from build123d import *

# Parameters (mm, degrees)
F0_R     = 38.1
F1_DEPTH = 2235.2
F2_R     = 38.1
F2_R_2   = 12.7
F3_DEPTH = 101.6
F4_R     = 38.1
F4_R_2   = 12.7
F5_DEPTH = 101.6


with BuildPart() as f1:
    # F0 (on Front) → F1 (new body)
    with BuildSketch(Plane.XZ):
        Circle(F0_R)
    extrude(amount=F1_DEPTH)

    # F2 (on face) → F3 (cut)
    with BuildSketch(Plane.XZ.offset(2235.2)):
        Circle(F2_R)
        Circle(F2_R_2, mode=Mode.SUBTRACT)
    extrude(amount=-F3_DEPTH, mode=Mode.SUBTRACT)

    # F4 (on face) → F5 (cut)
    with BuildSketch(Plane(origin=(0, 0, 0), x_dir=(-1, 0, 0), z_dir=(0, 1, 0))):
        Circle(F4_R)
        Circle(F4_R_2, mode=Mode.SUBTRACT)
    extrude(amount=-F5_DEPTH, mode=Mode.SUBTRACT)


solid = f1.part
The model under review builds one solid part; all positions refer to its coordinate system, in mm. A direction names the side the tool comes from. Give positions to 0.01 mm unless a question says otherwise; leave off trailing zeros. Order: outer loops, then holes, each group sorted by start corner. A loop starts at its lowest first (then second) coordinate and runs counter-clockwise, first axis right, second up. Notation, with made-up numbers: M 11.25,25 L 23.25,25 A26 cw 23.25,63 Z; hole C 86.5,-30 d10. An arc over 180 degrees is marked long. Answer in a Markdown table with one row per item. Add a question column.
1. Add section A-A on z = 0. State the section outline as (x, y) points.
2. Machinability: for faces 1 (the flat face through (16, -2133.6, 1)), 2 (the flat face through (-16, -101.6, 1)), 3 (the cylindrical face through (-30.235, -1103.376, -23.183)), which of the approach directions +Z, -Z, +X, -X, +Y, -Y give a long, thin tool a straight path to every point of the face, cutting with its end or side? Answer none if there is none.
3. Add section B-B on x = 0. State the section outline as (y, z) points.
4. For pin 1 Ø12 at (y, z) = (-1726.5, 7) entering from -X; pin 2 Ø1.5 at (x, z) = (-12, -17) entering from +Y; pin 3 Ø1.5 at (x, z) = (20, -30) entering from -Y, all flat-tipped, find the tip position at first contact; note any pin that passes through.
5. To check wall thickness, follow line 1 along Y through (x, z) = (-31, 21); line 2 along Z through (x, y) = (-4.5, -1016); line 3 along Z through (x, y) = (32, -1788). State the ranges of each line that lie inside material, in increasing order.
6. Add section C-C on y = -945.5. State the section outline as (x, z) points, plus the area to 3 significant figures.
The answers:
| question | item | result |
|---|---|---|
| 1 | outline | M -38.1,-2133.6 L -12.7,-2133.6 L -12.7,-2235.2 L 12.7,-2235.2 L 12.7,-2133.6 L 38.1,-2133.6 L 38.1,-101.6 L 12.7,-101.6 L 12.7,0 L -12.7,0 L -12.7,-101.6 L -38.1,-101.6 Z |
| 2 | face 1 | -Y |
| 2 | face 2 | +Y |
| 2 | face 3 | +Y, -Y |
| 3 | outline | M -2235.2,-12.7 L -2133.6,-12.7 L -2133.6,-38.1 L -101.6,-38.1 L -101.6,-12.7 L 0,-12.7 L 0,12.7 L -101.6,12.7 L -101.6,38.1 L -2133.6,38.1 L -2133.6,12.7 L -2235.2,12.7 Z |
| 4 | pin 1 | x = -38.09 |
| 4 | pin 2 | y = -101.6 |
| 4 | pin 3 | y = -2133.6 |
| 5 | line 1 | -2133.6 to -101.6 |
| 5 | line 2 | -37.83 to 37.83 |
| 5 | line 3 | -20.68 to 20.68 |
| 6 | outline | C 0,0 d76.2 |
| 6 | area | 4,560 mm2 |
